from build123d import *

# Parameters (mm, degrees)
F0_W     = 90
F0_H     = 80
F1_DEPTH = 70
F2_T     = -8
F3_R     = 5
F4_R     = 10
F5_R     = 30
F7_D     = 30
F9_D     = 22


with BuildPart() as f1:
    # F0 (on Front) → F1 (new body)
    with BuildSketch(Plane.XZ):
        Rectangle(F0_W, F0_H)
    extrude(amount=F1_DEPTH)

    # F2
    f2_openings = [f1.faces().sort_by_distance(p)[0] for p in [
        (0, -70, 0),
        (0, -35, 40),
        (0, -35, -40),
    ]]
    offset(amount=F2_T, openings=f2_openings)

    # F3
    f3_edges = [f1.edges().sort_by_distance(p)[0] for p in [
        (-37, -8, 0),
        (37, -8, 0),
    ]]
    fillet(f3_edges, radius=F3_R)

    # F4
    f4_edges = [f1.edges().sort_by_distance(p)[0] for p in [
        (-45, 0, 0),
        (45, 0, 0),
    ]]
    fillet(f4_edges, radius=F4_R)

    # F5
    f5_edges = [f1.edges().sort_by_distance(p)[0] for p in [
        (41, -70, 40),
        (-41, -70, 40),
        (41, -70, -40),
        (-41, -70, -40),
    ]]
    fillet(f5_edges, radius=F5_R)

    # F7 (through all)
    with Locations(Plane.XZ.offset(8)):
        with Locations((0, 0)):
            Hole(F7_D / 2)

    # F9 (through all)
    with Locations(Plane.YZ.offset(45)):
        with Locations((-35, 0)):
            Hole(F9_D / 2)


solid = f1.part
Verification items for the finished model (mm, model axes). A direction names the side the tool comes from. Give positions to 0.01 mm unless a question says otherwise; leave off trailing zeros. Order: outer loops, then holes, each group sorted by start corner. A loop starts at its lowest first (then second) coordinate and runs counter-clockwise, first axis right, second up. Notation, with made-up numbers: M 19.5,59.5 L 75.5,59.5 A23 ccw 75.5,79.5 Z; hole C 32.25,45 d5. An arc over 180 degrees is marked long. Use one line per item in the form item = value. Start each with the question number.
Q1. Access from +Z, -Z, +X, -X, +Y, -Y to the whole of each face (thin tool, end or side, straight path). Record for faces 1 (the cylindrical face through (36, -10, 1)), 2 (the cylindrical face through (-42.15, -3.01, 0.56)).
Q2. Section check D-D (y = -14.5). Enter the section's corners in (x, z).
Q3. Section check A-A (y = -35). Enter the section's corners in (x, z), then the cut area to 3 significant figures.
Q4. Go/stop test with flat-tipped pins: pin 1 Ø1 at (y, z) = (-8, 25) entering from -X; pin 2 Ø13 at (y, z) = (-35, 0) entering from +X; pin 3 Ø3 at (x, z) = (31, -3.5) entering from -Y. Record where each tip stops, or that it passes through.
Q5. Section check B-B (x = 0). Enter the section's corners in (y, z).
Q6. Scan lines: line 1 along X through (y, z) = (-28, -23.5); line 2 along Z through (x, y) = (-39, -35); line 3 along Z through (x, y) = (-38.5, -25). Record each from-to range of solid material in increasing order. Write a range as [from, to].
Q7. Mould release check, pull along Y, two halves, no side actions. Record for faces 3 (the cylindrical face through (-41.06, -26.27, -6.69)), 4 (the cylindrical face through (41.056, -60.979, 31.445)), 5 (the flat face through (-1, -6, 40)): +Y half, -Y half, draft (parallel to the pull), parting line (faces both ways), or undercut.
Q8. Section check C-C (z = 0). Enter the section's corners in (x, y), then the cut area to 3 significant figures.
Evaluation:
q1.face_1 = +Z, -Z, -Y
q1.face_2 = +Z, -Z, -X, +Y
q2.outline = M -45,-40 L -37,-40 L -37,40 L -45,40 Z; M 37,-40 L 45,-40 L 45,40 L 37,40 Z
q3.outline = M -45,-40 L -37,-40 L -37,-11 L -45,-11 Z; M -45,11 L -37,11 L -37,40 L -45,40 Z; M 37,-40 L 45,-40 L 45,-11 L 37,-11 Z; M 37,11 L 45,11 L 45,40 L 37,40 Z
q3.area = 928 mm2
q4.pin_1 = -44.89
q4.pin_2 = through
q4.pin_3 = -8.03
q5.outline = M -8,-40 L 0,-40 L 0,-15 L -8,-15 Z; M -8,15 L 0,15 L 0,40 L -8,40 Z
q6.line_1 = [-45, -37], [37, 45]
q6.line_2 = [-40, -11], [11, 40]
q6.line_3 = [-40, -4.58], [4.58, 40]
q7.face_3 = undercut
q7.face_4 = -Y half
q7.face_5 = draft
q8.outline = M -45,-70 L -37,-70 L -37,-46 L -45,-46 Z; M -45,-24 L -37,-24 L -37,-13 A5 cw -32,-8 L -15,-8 L -15,0 L -35,0 A10 ccw -45,-10 Z; M 15,-8 L 32,-8 A5 cw 37,-13 L 37,-24 L 45,-24 L 45,-10 A10 ccw 35,0 L 15,0 Z; M 37,-70 L 45,-70 L 45,-46 L 37,-46 Z
q8.area = 1,090 mm2
